Read the model definition and answer for the solid it produces. Units are mm, in the model's axes. Coordinates: 2 decimals unless noted, no trailing zeros. Loops run counter-clockwise (first coordinate to the right, second up) from the corner with the lowest first, then second, coordinate; pieces in that order, holes last. Notation, with made-up numbers: M 33,-9 L 51,-9 A21 cw 51,0 Z; hole C -27,12.25 d2. An arc over 180 degrees is marked long. Use one line per item in the form item = value. Start each with the question number.
1. Find the intervals of material crossed by probe 1 along Y at (x, z) = (-6.5, 4); probe 2 along Z at (x, y) = (-4, -79); probe 3 along Z at (x, y) = (22.5, -84.5), in increasing order. Write a range as [from, to].
2. The part is cut by section A-A (y = -75). Give the vertices of the cut face in (x, z).
3. The part is cut by section B-B (x = -3). Give the vertices of the cut face in (y, z), plus the area to 3 significant figures.
4. The part is cut by section C-C (z = 6.5). Give the vertices of the cut face in (x, y).
5. The part is cut by section D-D (x = 29.5). Give the vertices of the cut face in (y, z), plus the area to 3 significant figures.
6. Flat-ended cylindrical pins translate along their axes: pin 1 (4 mm diameter, centred on x = -17.5, y = -52.5, fed in from -Z); pin 2 (3.5 mm diameter, centred on x = -5, y = -2, fed in from +Z); pin 3 (2.5 mm diameter, centred on x = 12, y = -98.5, fed in from +Z); pin 4 (0.5 mm diameter, centred on y = -35, z = 0.5, fed in from +X). Find the tip coordinate at first contact, or state that the pin passes through.
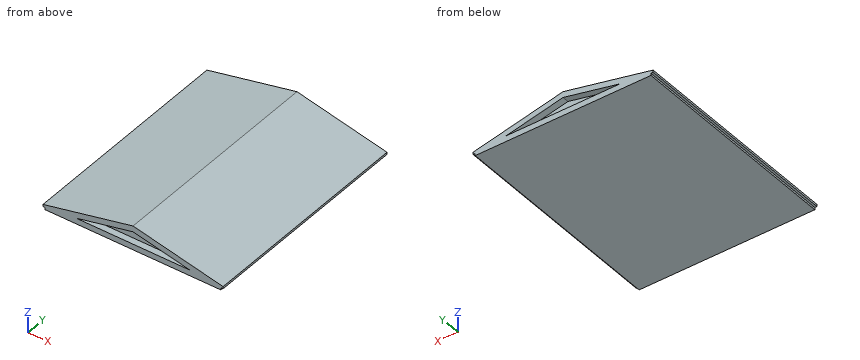
from build123d import *

# Parameters (mm, degrees)
F1_DEPTH = 100
F3_DEPTH = 3
F5_DEPTH = 3


with BuildPart() as f1:
    # F0 (on Front) → F1 (new body)
    with BuildSketch(Plane.XZ):
        Polygon((-40, 0), (0, 0), (40, 0), (40, 1), (41, 1), (41, 2), (0, 10.992676), (-41, 2), (-41, 1), (-40, 1), align=None)
    extrude(amount=F1_DEPTH)

    # F2 (on face) → F3 (cut)
    with BuildSketch(Plane(origin=(0, 0, 0), x_dir=(-1, 0, 0), z_dir=(0, 1, 0))):
        Polygon((0, 8.315965), (-25.994221, 2.61456), (0, 2.61456), align=None)
        Polygon((25.994221, 2.61456), (0, 8.315965), (0, 2.61456), align=None)
    extrude(amount=-F3_DEPTH, mode=Mode.SUBTRACT)

    # F4 (on face) → F5 (cut)
    with BuildSketch(Plane.XZ.offset(100)):
        Polygon((0, 2.61456), (25.994221, 2.61456), (0, 8.315965), (-25.994221, 2.61456), align=None)
    extrude(amount=-F5_DEPTH, mode=Mode.SUBTRACT)


solid = f1.part
Computed values:
q1.probe_1 = [-97, -3]
q1.probe_2 = [0, 10.12]
q1.probe_3 = [0, 6.06]
q2.outline = M -41,1 L -40,1 L -40,0 L 40,0 L 40,1 L 41,1 L 41,2 L 0,10.99 L -41,2 Z
q3.outline = M -100,0 L 0,0 L 0,2.61 L -3,2.61 L -3,7.66 L 0,7.66 L 0,10.33 L -100,10.33 L -100,7.66 L -97,7.66 L -97,2.61 L -100,2.61 Z
q3.area = 1,000 mm²
q4.outline = M -20.48,-100 L -8.28,-100 L -8.28,-97 L 8.28,-97 L 8.28,-100 L 20.48,-100 L 20.48,0 L 8.28,0 L 8.28,-3 L -8.28,-3 L -8.28,0 L -20.48,0 Z
q5.outline = M -100,0 L 0,0 L 0,4.52 L -100,4.52 Z
q5.area = 452 mm²
q6.pin_1 = 0
q6.pin_2 = 10.28
q6.pin_3 = 8.63
q6.pin_4 = 40
